from build123d import *

# Parameters (mm, degrees)
ESQUISSE1_W                     = 355.6
ESQUISSE1_H                     = 107.95
BOSS_EXTRU_1_DEPTH              = 6.35
ESQUISSE4_W                     = 6.35
ESQUISSE4_H                     = 10.16
ENL_V_MAT_EXTRU_3_DEPTH         = 6.35
R_P_TITION_LIN_AIRE2_COUNT      = 5
R_P_TITION_LIN_AIRE2_PITCH      = 20.32
R_P_TITION_LIN_AIRE2_COUNT_DIR2 = 2
R_P_TITION_LIN_AIRE2_PITCH_DIR2 = 349.25
ESQUISSE5_W                     = 25.4
ESQUISSE5_H                     = 6.35
ENL_V_MAT_EXTRU_4_DEPTH         = 6.35
R_P_TITION_LIN_AIRE3_COUNT      = 7
R_P_TITION_LIN_AIRE3_PITCH      = 50.8
ESQUISSE6_W                     = 12.7
ESQUISSE6_H                     = 6.35
ENL_V_MAT_EXTRU_5_DEPTH         = 6.35
ESQUISSE7_W                     = 25.4
ESQUISSE7_H                     = 6.35
ENL_V_MAT_EXTRU_6_DEPTH         = 6.35
R_P_TITION_LIN_AIRE5_COUNT      = 7
R_P_TITION_LIN_AIRE5_PITCH      = 50.8


with BuildPart() as part:
    # Esquisse1 → Boss.-Extru.1 (new body)
    with BuildSketch(Plane.XY):
        Rectangle(ESQUISSE1_W, ESQUISSE1_H)
    extrude(amount=BOSS_EXTRU_1_DEPTH)

    # Esquisse4 → Enlèv. mat.-Extru.3 (cut)
    with BuildSketch(Plane.XY.offset(6.35)):
        with Locations((-174.625, 38.735)):
            Rectangle(ESQUISSE4_W, ESQUISSE4_H)
    enl_v_mat_extru_3 = extrude(amount=-ENL_V_MAT_EXTRU_3_DEPTH, mode=Mode.SUBTRACT)

    # Répétition linéaire2: Enl_v. mat.-Extru.3 5 × 2
    with Locations(*[(j * R_P_TITION_LIN_AIRE2_PITCH_DIR2, -i * R_P_TITION_LIN_AIRE2_PITCH, 0) for i in range(R_P_TITION_LIN_AIRE2_COUNT) for j in range(R_P_TITION_LIN_AIRE2_COUNT_DIR2) if (i, j) != (0, 0)]):
        add(enl_v_mat_extru_3, mode=Mode.SUBTRACT)

    # Esquisse5 → Enlèv. mat.-Extru.4 (cut)
    with BuildSketch(Plane.XY.offset(6.35)):
        with Locations((-127, -50.8)):
            Rectangle(ESQUISSE5_W, ESQUISSE5_H)
    enl_v_mat_extru_4 = extrude(amount=-ENL_V_MAT_EXTRU_4_DEPTH, mode=Mode.SUBTRACT)

    # Répétition linéaire3: Enlèv. mat.-Extru.4 ×7
    with Locations(*[(i * R_P_TITION_LIN_AIRE3_PITCH, 0, 0) for i in range(1, R_P_TITION_LIN_AIRE3_COUNT)]):
        add(enl_v_mat_extru_4, mode=Mode.SUBTRACT)

    # Esquisse6 → Enlèv. mat.-Extru.5 (cut)
    with BuildSketch(Plane.XY.offset(6.35)):
        with Locations((-171.45, -50.8)):
            Rectangle(ESQUISSE6_W, ESQUISSE6_H)
    extrude(amount=-ENL_V_MAT_EXTRU_5_DEPTH, mode=Mode.SUBTRACT)

    # Esquisse7 → Enlèv. mat.-Extru.6 (cut)
    with BuildSketch(Plane.XY.offset(6.35)):
        with Locations((-152.4, 0)):
            Rectangle(ESQUISSE7_W, ESQUISSE7_H)
    enl_v_mat_extru_6 = extrude(amount=-ENL_V_MAT_EXTRU_6_DEPTH, mode=Mode.SUBTRACT)

    # Répétition linéaire5: Enlèv. mat.-Extru.6 ×7
    with Locations(*[(i * R_P_TITION_LIN_AIRE5_PITCH, 0, 0) for i in range(1, R_P_TITION_LIN_AIRE5_COUNT)]):
        add(enl_v_mat_extru_6, mode=Mode.SUBTRACT)


solid = part.part
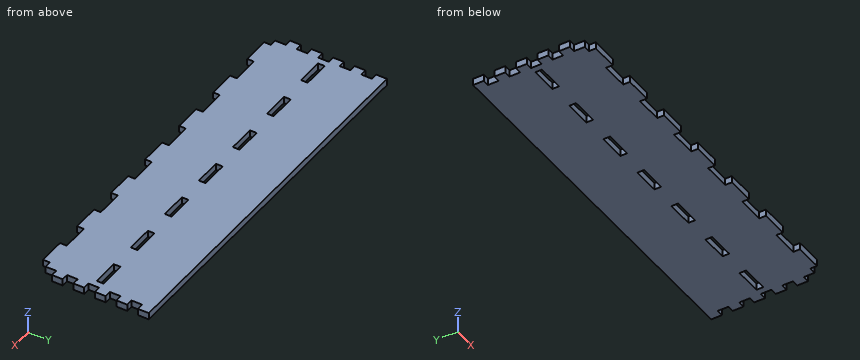
Read the model definition and answer for the solid it produces. Units are mm, in the model's axes. Give positions to 0.01 mm unless a question says otherwise; leave off trailing zeros. Loops run counter-clockwise (first coordinate to the right, second up) from the corner with the lowest first, then second, coordinate; pieces in that order, holes last. Notation, with made-up numbers: (-32, 82) -> (-20, 82) arc R25 ccw to (-20, 112) -> close; hole circle Ø7 at (62.25, -39.75). An arc over 180 degrees is marked (long way). Answer as CSV lines item,"result".
Item 1: Find section B-B on z = 4.5. State how many separate pieces and enclosed holes the cut face has, plus the area to 3 significant figures.
Returned:
separate pieces,"1"
enclosed holes,"7"
area,"35,500 mm²"
Item 2: Find section C-C on y = -22. Give the vertices of the cut face in (x, z), plus the area to 3 significant figures.
Returned:
outline,"(-171.45, 0) -> (171.45, 0) -> (171.45, 6.35) -> (-171.45, 6.35) -> close"
area,"2,180 mm²"
Item 3: Find section D-D on x = 32. Give the vertices of the cut face in (y, z) (3 decimals).
Returned:
outline,"(-47.625, 0) -> (53.975, 0) -> (53.975, 6.35) -> (-47.625, 6.35) -> close"
Item 4: Find section A-A on x = 149. Give the vertices of the cut face in (y, z) (3 decimals), plus the area to 3 significant figures.
Returned:
outline,"(-53.975, 0) -> (-3.175, 0) -> (-3.175, 6.35) -> (-53.975, 6.35) -> close; (3.175, 0) -> (53.975, 0) -> (53.975, 6.35) -> (3.175, 6.35) -> close"
area,"645 mm²"
Item 5: Each of these flat-tipped pins is pushed along its axis until it touches: pin 1 (1.9 mm diameter, centred on y = 0.5, z = 2.5, fed in from +X); pin 2 (1.5 mm diameter, centred on y = 15.5, z = 4.5, fed in from -X); pin 3 (3 mm diameter, centred on y = -49.5, z = 4, fed in from -X). Where does it stop, or does it pass through?
Returned:
pin 1,"stops at x = 171.45"
pin 2,"stops at x = -171.45"
pin 3,"stops at x = -165.1"
Item 6: Consider line 1 (Y direction, x = 3, z = 6) (3 decimals); line 2 (Y direction, x = 29, z = 2.75) (3 decimals); line 3 (X direction, y = 39, z = 3.25). Determine where each line is inside the solid, lowest interval first. Write a range as [from, to].
Returned:
line 1,"y = [-53.975, -3.175], [3.175, 53.975]"
line 2,"y = [-47.625, 53.975]"
line 3,"x = [-171.45, 171.45]"
